Geometry check sheet. Reference: drawing and pictorial views, mm from the part's lowest x, y, z. Give positions to 0.01 mm unless a question says otherwise; leave off trailing zeros. Write each loop counter-clockwise with the first axis right and the second up, starting at its lowest first coordinate (ties: lowest second). Pieces come first, ordered by that corner, then holes. Notation, with made-up numbers: (4.5, -29) - (8.5, -29) arc R21 ccw to (8.5, -13) - close; hole circle Ø4 at (33.5, -3.5). An arc over 180 degrees is marked (long way). Write item = value, one per line. Start each with the question number.
(1) Section check D-D, the plane x = 5. Enter the section's corners in (y, z).
(2) Section check C-C, the plane y = 29.5. Enter the section's corners in (x, z).
(3) Thickness scan on L1, parallel to Z at x = 64, y = 32; L2, parallel to X at y = 32, z = 4; L3, parallel to X at y = 15, z = 3.5. Record the ranges inside material, lowest first.
(4) Depth check by flat-ended pin: pin 1 Ø3 at (x, z) = (64, 5) entering from -Y. Enter the tip coordinate at first touch or a pass-through.
(5) Section check B-B, the plane x = 64. Enter the section's corners in (y, z), plus the area to 3 significant figures.
(6) Section check A-A, the plane z = 5. Enter the section's corners in (x, y), plus the area to 3 significant figures.
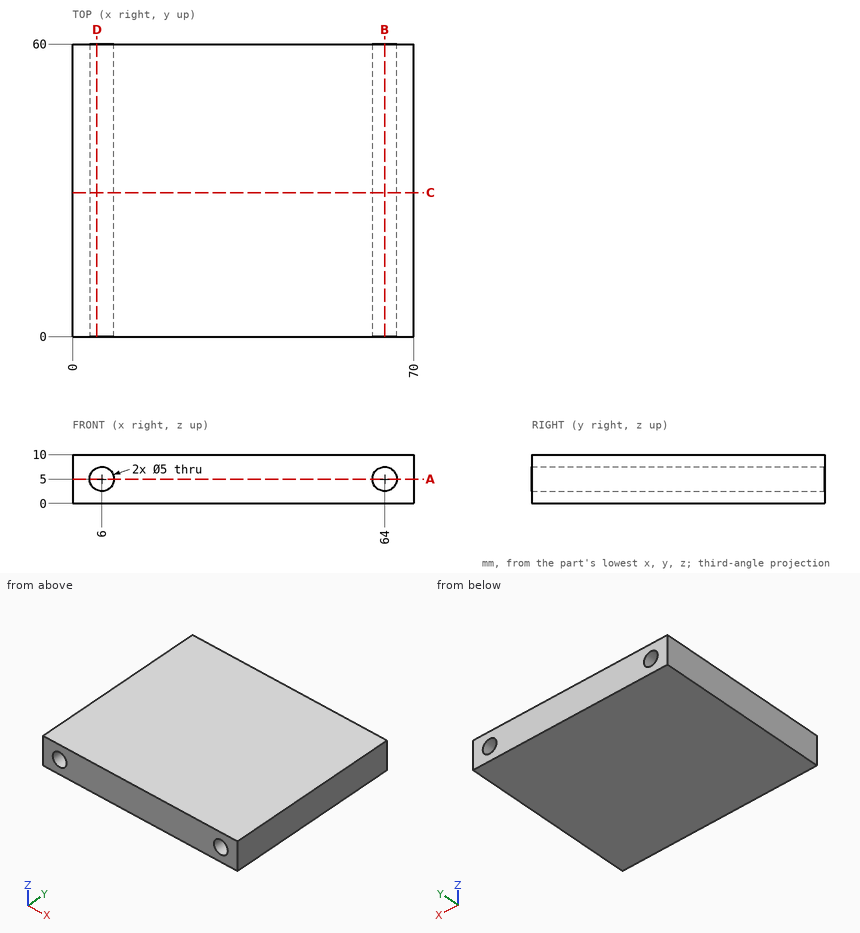
Model answer:
q1.outline = (0, 0) - (60, 0) - (60, 2.71) - (0, 2.71) - close; (0, 7.29) - (60, 7.29) - (60, 10) - (0, 10) - close
q2.outline = (0, 0) - (70, 0) - (70, 10) - (0, 10) - close; hole circle Ø5 at (6, 5); hole circle Ø5 at (64, 5)
q3.L1 = 0 to 2.5, 7.5 to 10
q3.L2 = 0 to 3.71, 8.29 to 61.71, 66.29 to 70
q3.L3 = 0 to 4, 8 to 62, 66 to 70
q4.pin_1 = through
q5.outline = (0, 0) - (60, 0) - (60, 2.5) - (0, 2.5) - close; (0, 7.5) - (60, 7.5) - (60, 10) - (0, 10) - close
q5.area = 300 mm²
q6.outline = (0, 0) - (3.5, 0) - (3.5, 60) - (0, 60) - close; (8.5, 0) - (61.5, 0) - (61.5, 60) - (8.5, 60) - close; (66.5, 0) - (70, 0) - (70, 60) - (66.5, 60) - close
q6.area = 3,600 mm²
